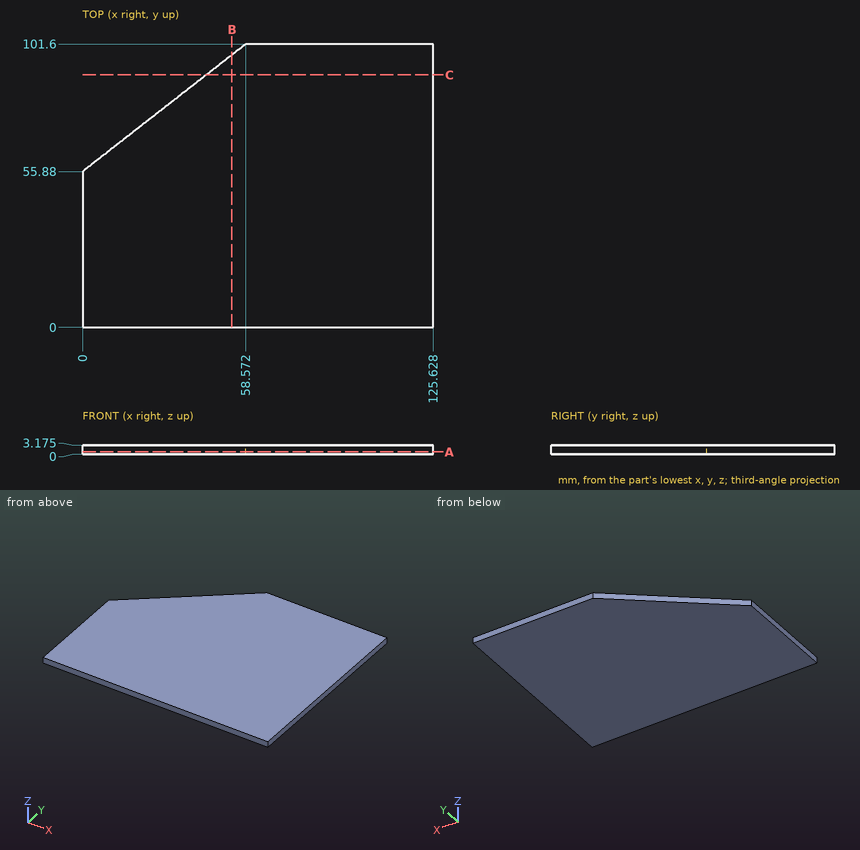
Can you work these out from the drawing? Everything is in mm from the part's minimum corner. Give positions to 0.01 mm unless a question says otherwise; leave off trailing zeros. Loops run counter-clockwise (first coordinate to the right, second up) from the corner with the lowest first, then second, coordinate; pieces in that order, holes last. Notation, with made-up numbers: (4.25, 50.25) - (58.25, 50.25) arc R4 ccw to (58.25, 57.25) - close; hole circle Ø3 at (50, -34). An arc over 180 degrees is marked (long way). Use one line per item in the form item = value.
1. I want a section at B-B (x = 53.5). Please give me the cut outline in (y, z) (1 decimal), and give its area (3 significant figures).
Response values:
outline = (0, 0) - (97.6, 0) - (97.6, 3.2) - (0, 3.2) - close
area = 310 mm²
2. I want a section at C-C (y = 90.5). Please give me the cut outline in (x, z) (1 decimal), and give its area (3 significant figures).
Response values:
outline = (44.4, 0) - (125.6, 0) - (125.6, 3.2) - (44.4, 3.2) - close
area = 258 mm²
3. I need wall thicknesses on probe 1 along X at (y, z) = (97, 0.9); probe 2 along X at (y, z) = (88.5, 1.7); probe 3 along Y at (x, z) = (29, 2.15) (1 decimal). Which ranges of each line are inside material? Lowest first, please.
Response values:
probe_1 = 52.68 to 125.63
probe_2 = 41.79 to 125.63
probe_3 = 0 to 78.5
4. I want a section at A-A (z = 0.9). Please give me the cut outline in (x, y).
Response values:
outline = (0, 0) - (125.63, 0) - (125.63, 101.6) - (58.57, 101.6) - (0, 55.88) - close
